For this review, take the finished solid that the model builds, in its own axes (mm). Face numbers are marked on the shaded views. Coordinates: 2 decimals unless noted, no trailing zeros. Write each loop counter-clockwise with the first axis right and the second up, starting at its lowest first coordinate (ties: lowest second). Pieces come first, ordered by that corner, then holes. Notation, with made-up numbers: M -31,84.5 L 25,84.5 A29 ccw 25,121.5 Z; hole C 7,73 d2. An arc over 180 degrees is marked long. One line per question, with ' | ' between items.
Autodesk Inventor part; units mm, degrees
ref_plane "YZ Plane" through (0, 0, 0) normal (1, 0, 0) x (0, 1, 0)
ref_plane "XZ Plane" through (0, 0, 0) normal (0, 1, 0) x (-1, 0, 0)
ref_plane "XY Plane" through (0, 0, 0) normal (0, 0, 1) x (1, 0, 0)
sketch "Sketch1" plane through (0, 0, 0) normal (0, 0, 1) x (1, 0, 0)
  circle A0 centre (0, 0) radius 10.16
  dimension "d0" = 20.32
extrude "Extrusion1" add sketch "Sketch1" against normal blind 25.4
sketch "Sketch2" plane through (0, 0, 0) normal (0, 0, 1) x (1, 0, 0)
  circle A0 centre (0, 0) radius 9.144
  dimension "d3" = 18.288
extrude "Extrusion2" cut sketch "Sketch2" against normal blind 10.668
sketch "Sketch3" plane through (0, 0, -25.4) normal (0, 0, -1) x (-1, 0, 0)
  circle A0 centre (0, 0) radius 2.667
  line L0 (2.159, 1.5658) -> (2.159, -1.5658)
  dimension "d6" = 5.334
  dimension "d7" = 4.826
extrude "Extrusion3" cut sketch "Sketch3" against normal blind 11.43 contours L0 A0 picked at (-0.0356, -0.8771)
sketch "Sketch4" plane through (0, 0, -25.4) normal (0, 0, -1) x (-1, 0, 0)
  circle A0 centre (0, 0) radius 3.81
  circle A1 centre (0, 0) radius 10.16
  dimension "d10" = 7.62
extrude "Extrusion4" cut sketch "Sketch4" against normal blind 11.43
fillet "Fillet2" radius 3.175 1 edges at (-10.16, 0, -13.97)
sketch "Sketch6" plane through (0, 0, 0) normal (0, 0, 1) x (1, 0, 0)
  line L0 (-10.922, -1.27) -> (-5.08, -1.27)
  line L1 (-5.08, -1.27) -> (-5.08, 1.27)
  line L2 (-5.08, 1.27) -> (-10.922, 1.27)
  line L3 (-10.922, 1.27) -> (-10.922, -1.27)
  point P0 (0, 0)
  dimension "d19" = 2.54
  dimension "d20" = 5.08
  dimension "d21" = 1.27
extrude "Extrusion6" cut sketch "Sketch6" against normal blind 10.668
sketch "Sketch7" plane through (0, 0, 0) normal (0, 0, 1) x (1, 0, 0)
  arc A0 (-9.0554, -1.27) -> (-9.0554, 1.27) centre (0, 0) ccw
  circle A1 centre (0, -9.144) radius 0.254
  dimension "d24" = 0.508
extrude "Extrusion7" add sketch "Sketch7" against normal blind 10.668
pattern_circular "Circular Pattern1" count 35 over 360 about axis through (0, 0, 0) along (0, 0, -1) of "Extrusion7"
sketch "Sketch8" plane through (0, 0, 0) normal (0, 0, 1) x (1, 0, 0)
  line L0 (-10.7775, -1.27) -> (-8.1519, -1.27)
  line L1 (-8.1519, -1.27) -> (-8.1519, 1.2704)
  line L2 (-8.1519, 1.2704) -> (-10.7775, 1.2704)
  line L3 (-10.7775, 1.2704) -> (-10.7775, -1.27)
  point P0 (0, 0)
extrude "Extrusion8" cut sketch "Sketch8" against normal blind 10.668
sketch "Sketch9" plane through (0, 0, 0) normal (0, 0, 1) x (1, 0, 0)
  circle A0 centre (0, 0) radius 9.144
  line L0 (-9.2823, -1.8753) -> (-8.4046, -1.8753)
  line L1 (-8.4046, -1.8753) -> (-8.4046, -0.367)
  line L2 (-8.4046, -0.367) -> (-9.2823, -0.367)
  line L3 (-9.2823, -0.367) -> (-9.2823, -1.8753)
  point P0 (-9.1366, -0.367)
  point P1 (-8.9496, -1.8753)
extrude "Extrusion9" cut sketch "Sketch9" against normal blind 10.668 contours L2 L1 L0 A0 picked at (-8.6163, -1.2062)
properties part number "Coupler2"
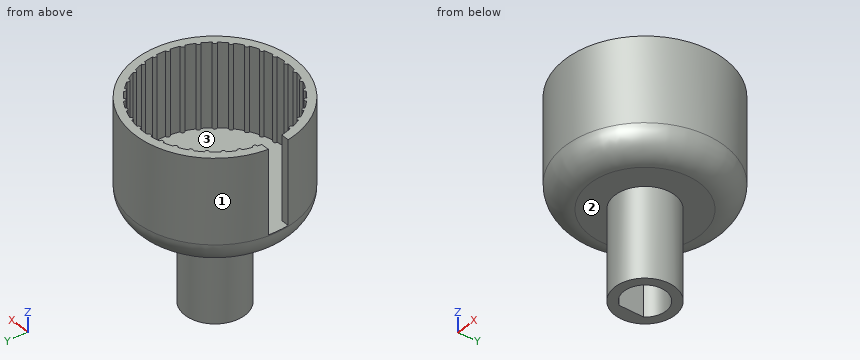
1. For line 1 along Y through (x, z) = (0, -20.75); line 2 along X through (y, z) = (1, -15.5); line 3 along X through (y, z) = (4, -5), list the stretches that pass through material, from the lowest coordinate up.
Computed values:
line 1: y = -3.81 to -2.67, 2.67 to 3.81 | line 2: x = -3.68 to -2.16, 2.47 to 3.68 | line 3: x = -9.34 to -8.22, 8.22 to 9.34
2. Clearance check with flat-ended pins moving along their axes: P1, Ø6, axis at x = 5.5, y = 0.5, coming from the +Z side; P2, Ø5, axis at x = -7, y = -6.5, coming from the -Z side; P3, Ø0.5, axis at x = -9.5, z = -8, coming from the +Y side. State where each tip first meets the part, or that it passes through.
Computed values:
P1: stops at z = -10.67 | P2: stops at z = -13.97 | P3: stops at y = 4.2
3. Draft analysis for pull direction X (two halves, no side actions). For the marked faces 1, 2 and 3, state which applies: pulls with the +X half, pulls with the -X half, needs draft (parallel to the pull), parting line crosses it, or undercut.
Computed values:
face 1: parting line crosses it | face 2: needs draft | face 3: undercut
4. Take a section at A-A on z = -23.5. State the section outline as (x, y) points.
Computed values:
outline: C 0,0 d7.62; hole M -2.16,-1.57 A2.67 ccw long -2.16,1.57 Z
